The listing builds one solid part. Answer for the finished solid, in the listing's coordinates (mm). A direction names the side the tool comes from. Give positions to 0.01 mm unless a question says otherwise; leave off trailing zeros. Order: outer loops, then holes, each group sorted by start corner. A loop starts at its lowest first (then second) coordinate and runs counter-clockwise, first axis right, second up.
```python
from build123d import *

# Parameters (mm, degrees)
EXTRUDE_1_DEPTH = 11.6
EXTRUDE_2_DEPTH = 3.5
SKETCH_3_R      = 1
EXTRUDE_3_DEPTH = 1
SKETCH_3_3_R    = 1
SKETCH_3_3_R_2  = 2.8
EXTRUDE_4_DEPTH = 0.4
SKETCH_5_R      = 2
EXTRUDE_5_DEPTH = 3.2


with BuildPart() as part:
    # ｽｹｯﾁ1 → ﾎﾞｽ - 押し出し1 (new body)
    with BuildSketch(Plane(origin=(0, 0, 0), x_dir=(1, 0, 0), z_dir=(0, 1, 0))):
        Polygon((0, 0), (18.6, 0), (23.8, 2.764889045), (23.8, 20.8), (0, 20.8), align=None)
    extrude(amount=EXTRUDE_1_DEPTH)

    # ｽｹｯﾁ2 → ﾎﾞｽ - 押し出し2 (add)
    with BuildSketch(Plane(origin=(0, 0, -20.8), x_dir=(-1, 0, 0), z_dir=(0, 0, -1))):
        with BuildLine():
            Line((-14.08660724, 9.6), (-12, 8.8))
            ThreePointArc((-12, 8.8), (-9, 5.8), (-12, 2.8))
            Line((-12, 2.8), (-14.08660724, 2))
            ThreePointArc((-14.08660724, 2), (-23.8, 5.8), (-14.08660724, 9.6))
        make_face()
    extrude(amount=EXTRUDE_2_DEPTH)

    # ｽｹｯﾁ3 → ﾎﾞｽ - 押し出し3 (add)
    with BuildSketch(Plane(origin=(0, 0, -24.3), x_dir=(-1, 0, 0), z_dir=(0, 0, -1))):
        with Locations((-11.2, 5.8)):
            Circle(SKETCH_3_R)
    extrude(amount=EXTRUDE_3_DEPTH)

    # ｽｹｯﾁ3<3> → ﾎﾞｽ - 押し出し4 (add)
    with BuildSketch(Plane(origin=(0, 0, -24.3), x_dir=(-1, 0, 0), z_dir=(0, 0, -1))):
        with Locations((-11.2, 5.8)):
            Circle(SKETCH_3_3_R)
        with Locations((-18.2, 5.8)):
            Circle(SKETCH_3_3_R_2)
    extrude(amount=EXTRUDE_4_DEPTH)

    # ｽｹｯﾁ5 → ﾎﾞｽ - 押し出し5 (add)
    with BuildSketch(Plane(origin=(0, 0, -24.7), x_dir=(-1, 0, 0), z_dir=(0, 0, -1))):
        with Locations((-18.2, 5.8)):
            Circle(SKETCH_5_R)
    extrude(amount=EXTRUDE_5_DEPTH)


solid = part.part
```
1) For a pull along X with two mould halves and no side action, classify faces 1 (the flat face through (23.8, 6, -12)), 2 (the flat face through (13.029, 2.406, -22.526)), 3 (the cylindrical face through (10.246, 6.1, -24.793)), 4 (the flat face through (12, 11.6, -11)) as +X half, -X half, draft (parallel to the pull), parting line (faces both ways), or undercut.
Geometry says:
face 1: +X half
face 2: -X half
face 3: undercut
face 4: draft
2) Find section B-B (z = -23.75). Write down the section's boundary in (x, y), then the cut area to 3 significant figures.
Geometry says:
outline: (12, 2.8) - (14.09, 2) arc R5.6 ccw (long way) to (14.09, 9.6) - (12, 8.8) arc R3 ccw to start
area: 119 mm2
3) A tool of negligible diameter and unlimited length cuts with its end or side. For faces 5 (the flat face through (11, 6, -25.3)), 6 (the cylindrical face through (9, 5.9, -22.5)), 7 (the cylindrical face through (23.797, 5.612, -22.526)), 8 (the flat face through (13.058, 9.206, -22.526)), from which of +Z, -Z, +X, -X, +Y, -Y can it reach the whole face along a straight path? Write none if from no direction.
Geometry says:
face 5: -Z, -X, +Y, -Y
face 6: -Z, -X
face 7: -Z
face 8: -Z, -X, +Y
4) Find section D-D (x = 19). Write down the section's boundary in (y, z), then the cut area to 3 significant figures.
Geometry says:
outline: (0, -20.8) - (0.26, -20.8) - (0.26, -24.3) - (3.12, -24.3) - (3.12, -24.7) - (3.97, -24.7) - (3.97, -27.9) - (7.63, -27.9) - (7.63, -24.7) - (8.48, -24.7) - (8.48, -24.3) - (11.34, -24.3) - (11.34, -20.8) - (11.6, -20.8) - (11.6, -0.21) - (0, -0.21) - close
area: 291 mm2
5) Given P1, Ø5, axis at x = 4, y = 6.5, coming from the -Z side; P2, Ø1.6, axis at x = 11.5, y = 5.5, coming from the -Z side, each flat-ended and moving along its own axis, determine where each tip first touches the part or whether it passes through.
Geometry says:
P1: stops at z = -20.8
P2: stops at z = -25.3
6) Find section A-A (x = 11.2). Write down the section's boundary in (y, z), then the cut area to 3 significant figures.
Geometry says:
outline: (0, -20.8) - (2.91, -20.8) - (2.91, -24.3) - (4.8, -24.3) - (4.8, -25.3) - (6.8, -25.3) - (6.8, -24.3) - (8.69, -24.3) - (8.69, -20.8) - (11.6, -20.8) - (11.6, 0) - (0, 0) - close
area: 264 mm2
7) Find section C-C (x = 22). Write down the section's boundary in (y, z).
Geometry says:
outline: (0, -20.8) - (1.69, -20.8) - (1.69, -24.3) - (9.91, -24.3) - (9.91, -20.8) - (11.6, -20.8) - (11.6, -1.81) - (0, -1.81) - close
8) Straight lines are drawn through the part: probe 1 along Z at (x, y) = (11.5, 7.5); probe 2 along Z at (x, y) = (11.25, 0.5); probe 3 along X at (y, z) = (7.5, -23). For each, find the intervals that lie inside material, in ascending order.
Geometry says:
probe 1: z = -24.3 to 0
probe 2: z = -20.8 to 0
probe 3: x = 9.53 to 23.54
